Geometry check sheet. Reference: the model listing, model coordinates, mm. Face numbers are marked on the shaded views. A direction names the side the tool comes from. Round coordinates to 2 decimals unless told otherwise and drop trailing zeros. Write each loop counter-clockwise with the first axis right and the second up, starting at its lowest first coordinate (ties: lowest second). Pieces come first, ordered by that corner, then holes. Notation, with made-up numbers: M 84,23.25 L 119,23.25 A24 ccw 119,36.25 Z; hole C 63.5,22.25 d1. An arc over 180 degrees is marked long. One line per item, written item: value. Start each with the question number.
1. Access from +Z, -Z, +X, -X, +Y, -Y to the whole of each face (thin tool, end or side, straight path). Record for the marked faces 1 and 2.
2. Depth check by flat-ended pin: P1, Ø8, axis at y = 26, z = 2.5, coming from the -X side; P2, Ø4, axis at x = -18.125, y = 30.175, coming from the -Z side; P3, Ø10, axis at x = -10, y = 15, coming from the -Z side. Enter the tip coordinate at first touch or a pass-through.
3. Section check D-D (x = -15.5). Record the boundary of the cut face in (y, z).
4. Scan lines: probe 1 along Y at (x, z) = (-15.7, 8.9); probe 2 along X at (y, z) = (3, 1); probe 3 along Z at (x, y) = (11, 23). Record each from-to range of solid material in increasing order. Write a range as [from, to].
5. Section check C-C (x = 3.5). Record the boundary of the cut face in (y, z), and give its area (3 significant figures).
6. Release check for a two-part mould opening along X. For the marked faces 3, 4, 5 and 6 record: pulls with the +X half, pulls with the -X half, needs draft (parallel to the pull), parting line crosses it, or undercut.
7. Section check B-B (z = 0). Record the boundary of the cut face in (x, y), and give its area (4 significant figures).
8. Section check A-A (y = 36.25). Record the boundary of the cut face in (x, z).
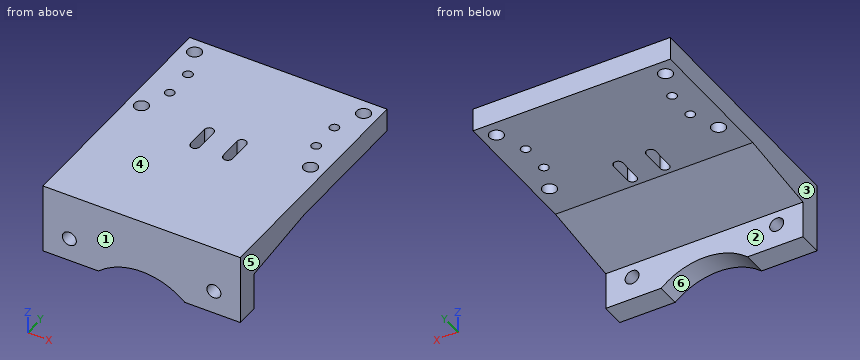
Autodesk Fusion 360 part; units mm, degrees
sketch "Sketch1" plane through (0, 0, 0) normal (0, 1, 0) x (1, 0, 0)
  line L0 (-21.15, 5) -> (21.15, 5)
  line L1 (21.15, 5) -> (21.15, -10)
  line L2 (21.15, -10) -> (-21.15, -10)
  line L3 (-21.15, -10) -> (-21.15, 5)
  line L4 (-15.5, 0) -> (15.5, 0) construction
  circle A0 centre (-15.5, 0) radius 1.5
  circle A1 centre (15.5, 0) radius 1.5
  circle A2 centre (0, 15.5) radius 14
  dimension "d1" = 42.3
  dimension "d2" = 15
  dimension "d3" = 31
  dimension "d4" = 5.65
  dimension "d5" = 3
  dimension "d6" = 3
  dimension "d9" = 28
  dimension "d13" = 15.5
  dimension "d14" = 5
extrude "Extrude1" add sketch "Sketch1" along normal blind 5 contours L0 L1 L2 L3 A2
sketch "Sketch2" plane through (0, 5, 0) normal (0, 1, 0) x (-1, 0, 0)
  line L0 (21.15, 5) -> (-21.15, 5)
  line L1 (-21.15, 5) -> (-21.15, 10)
  line L2 (-21.15, 10) -> (21.15, 10)
  line L3 (21.15, 10) -> (21.15, 5)
  circle A0 centre (-15.5, 0) radius 1.5
  circle A1 centre (15.5, 0) radius 1.5
  line L4 (-21.15, 10) -> (-21.15, -5)
  line L5 (-21.15, -5) -> (-9.2601, -5)
  arc A2 (9.2601, -5) -> (-9.2601, -5) centre (0, -15.5) ccw
  line L6 (9.2601, -5) -> (21.15, -5)
  line L7 (21.15, -5) -> (21.15, 10)
  line L8 (21.15, 10) -> (-21.15, 10)
  dimension "d22" = 5
  dimension "d23" = 42.3
extrude "Extrude2" add sketch "Sketch2" along normal blind 47.5 contours L0 L1 L2 L3 L4 L7 L8
sketch "Sketch3" plane through (0, 0, 5) normal (0, 0, -1) x (-1, 0, 0)
  line L0 (-15.7, 42.75) -> (-15.7, 36.25) construction
  circle A0 centre (-15.7, 42.75) radius 1
  circle A1 centre (-15.7, 36.25) radius 1
  line L1 (-21.15, 52.5) -> (21.15, 52.5)
  line L2 (0, 52.5) -> (0, 12.5) construction
  line L3 (-4.5, 30) -> (-4.5, 25)
  arc A2 (-4.5, 25) -> (-2.5, 25) centre (-3.5, 25) ccw
  line L4 (-2.5, 25) -> (-2.5, 30)
  arc A3 (-2.5, 30) -> (-4.5, 30) centre (-3.5, 30) ccw
  line L5 (-3.5, 30) -> (-3.5, 25) construction
  dimension "d26" = 6.5
  dimension "d27" = 2
  dimension "d28" = 2
  dimension "d30" = 5.45
  dimension "d32" = 2
  dimension "d33" = 5
  dimension "d34" = 3.5
  dimension "d35" = 25
  dimension "d51" = 42.75
extrude "Extrude3" cut sketch "Sketch3" against normal through all
mirror "Mirror1" about plane through (0, 0, 0) normal (1, 0, 0) of "Extrude3"
sketch "Sketch4" plane through (0, 0, 5) normal (0, 0, -1) x (-1, 0, 0)
  circle A0 centre (15.7, 42.75) radius 1
  circle A1 centre (15.7, 36.25) radius 1
  circle A2 centre (-15.7, 42.75) radius 1
  circle A3 centre (-15.7, 36.25) radius 1
  circle A4 centre (15.7, 42.75) radius 2.5
  circle A5 centre (15.7, 36.25) radius 1
  circle A6 centre (15.7, 36.25) radius 2.5
  circle A7 centre (-15.7, 42.75) radius 2.5
  circle A8 centre (-15.7, 36.25) radius 2.5
  dimension "d37" = 5
  dimension "d38" = 5
  dimension "d39" = 5
  dimension "d40" = 5
chamfer "Chamfer1" distance 2 distance2 18 1 edges at (0, 5, 5) measured on face at (0, 5, 2.8333)
sketch "Sketch5" plane through (0, 0, 10) normal (0, 0, 1) x (1, 0, 0)
  line L0 (-18.125, 49.175) -> (-18.125, 30.175)
  circle A0 centre (-18.125, 49.175) radius 1.5
  circle A1 centre (-18.125, 30.175) radius 1.5
  line L1 (-21.15, 0) -> (-21.15, 52.5)
  circle A2 centre (-15.7, 42.75) radius 1
  dimension "d45" = 19
  dimension "d46" = 3
  dimension "d47" = 3
  dimension "d49" = 6.425
  dimension "d50" = 2.425
extrude "Extrude5" cut sketch "Sketch5" against normal through all contours A1 | A0
mirror "Mirror2" about plane through (0, 0, 0) normal (1, 0, 0) of "Extrude5"
Result sheet:
1. face 1: +Z, -Z, +X, -X, -Y
1. face 2: -Z, +X, -X, +Y
2. P1: stops at x = -21.15
2. P2: stops at z = 5
2. P3: stops at z = 3.56
3. outline: M 0,-5 L 5,-5 L 5,-1.5 L 0,-1.5 Z; M 0,1.5 L 5,1.5 L 5,3 L 23,5 L 35.27,5 L 35.27,10 L 0,10 Z; M 37.23,5 L 41.77,5 L 41.77,10 L 37.23,10 Z; M 43.73,5 L 52.5,5 L 52.5,10 L 43.73,10 Z
4. probe 1: y = [0, 35.25], [37.25, 41.75], [43.75, 52.5]
4. probe 2: x = [-21.15, -16.62], [-14.38, 14.38], [16.62, 21.15]
4. probe 3: z = [5, 10]
5. outline: M 0,-1.94 L 5,-1.94 L 5,3 L 23,5 L 24,5 L 24,10 L 0,10 Z; M 31,5 L 52.5,5 L 52.5,10 L 31,10 Z
5. area: 280 mm2
6. face 3: pulls with the -X half
6. face 4: needs draft
6. face 5: pulls with the +X half
6. face 6: undercut
7. outline: M -21.15,0 L -17,0 L -17,5 L -21.15,5 Z; M -14,0 L 14,0 L 14,5 L -14,5 Z; M 17,0 L 21.15,0 L 21.15,5 L 17,5 Z
7. area: 181.5 mm2
8. outline: M -21.15,5 L -16.7,5 L -16.7,10 L -21.15,10 Z; M -14.7,5 L 14.7,5 L 14.7,10 L -14.7,10 Z; M 16.7,5 L 21.15,5 L 21.15,10 L 16.7,10 Z
